Build history of the part. All positions in model axes, mm. Face numbers are marked on the shaded views. Coordinates: 2 decimals unless noted, no trailing zeros. Write each loop counter-clockwise with the first axis right and the second up, starting at its lowest first coordinate (ties: lowest second). Pieces come first, ordered by that corner, then holes.
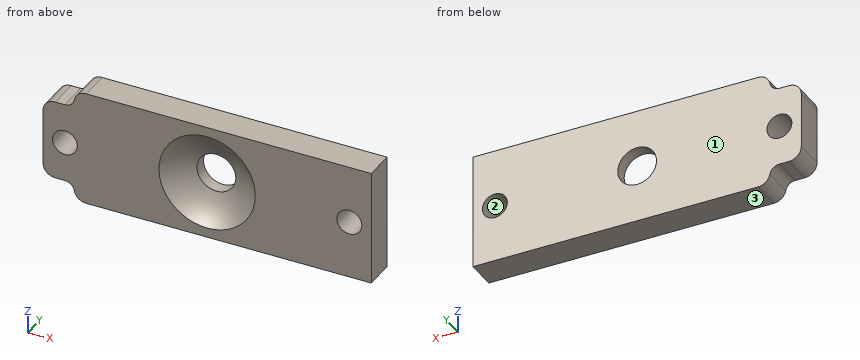
```python
from build123d import *

# Parameters (mm, degrees)
SKETCH2_W           = 68.58
SKETCH2_H           = 24.13
SKETCH2_R           = 2.6
BOSS_EXTRUDE1_DEPTH = 6.35
CUT_EXTRUDE1_DEPTH  = 7.35
FILLET3_R           = 2.54
SKETCH4_R           = 4.05
CUT_EXTRUDE2_DEPTH  = 7.3500001


with BuildPart() as part:
    # Sketch2 → Boss-Extrude1 (new body)
    with BuildSketch(Plane(origin=(0, 0, 0), x_dir=(1, 0, 0), z_dir=(0, 1, 0))):
        with Locations((34.29, 12.065)):
            Rectangle(SKETCH2_W, SKETCH2_H)
        with Locations((4.57, 12.065)):
            Circle(SKETCH2_R, mode=Mode.SUBTRACT)
        with Locations((64.01, 12.065)):
            Circle(SKETCH2_R, mode=Mode.SUBTRACT)
    extrude(amount=BOSS_EXTRUDE1_DEPTH)

    # Sketch3 → Cut-Extrude1 (cut, through all)
    with BuildSketch(Plane(origin=(0, 6.35, 0), x_dir=(1, 0, 0), z_dir=(0, 1, 0))):
        with BuildLine():
            Line((4.57, 3.715), (0, 3.715))
            Line((0, 3.715), (0, 0))
            Line((0, 0), (6.57, 0))
            Line((6.57, 0), (6.57, 1.715))
            ThreePointArc((6.57, 1.715), (5.984213562, 3.129213562), (4.57, 3.715))
        make_face()
        with BuildLine():
            ThreePointArc((4.57, 20.415), (5.984213562, 21.000786438), (6.57, 22.415))
            Line((6.57, 22.415), (6.57, 24.13))
            Line((6.57, 24.13), (0, 24.13))
            Line((0, 24.13), (0, 20.415))
            Line((0, 20.415), (4.57, 20.415))
        make_face()
    extrude(amount=-CUT_EXTRUDE1_DEPTH, mode=Mode.SUBTRACT)

    # Fillet3
    fillet3_edges = [part.edges().sort_by_distance(p)[0] for p in [
        (6.57, 3.175, 0),
        (0, 3.175, -3.715),
        (0, 3.175, -20.415),
        (6.57, 3.175, -24.13),
    ]]
    fillet(fillet3_edges, radius=FILLET3_R)

    # Sketch4 → Cut-Extrude2 (cut, through all)
    with BuildSketch(Plane(origin=(0, 6.35, 0), x_dir=(1, 0, 0), z_dir=(0, 1, 0))):
        with Locations((34.29, 12.065)):
            Circle(SKETCH4_R)
    extrude(amount=-CUT_EXTRUDE2_DEPTH, mode=Mode.SUBTRACT)

    # Sketch8 one side → Cut-Revolve6 (revolve, cut)
    with BuildSketch(Plane(origin=(34.29, 0, 0), x_dir=(0, 0, -1), z_dir=(1, 0, 0))):
        with BuildLine():
            Line((12.065, 0), (22.13, 0))
            ThreePointArc((22.13, 0), (17.5473974, 3.215969501), (12.065, 4.35))
            Line((12.065, 4.35), (12.065, 0))
        make_face()
    revolve(axis=Axis((34.29, 6.35, -12.065), (0, -1, 0)), mode=Mode.SUBTRACT)


solid = part.part
```
1. Probe line 1 along X through (y, z) = (6, -12); line 2 along X through (y, z) = (5, -12.75); line 3 along Z through (x, y) = (34.29, 5.3) (3 decimals). List the from-to ranges inside material, lowest first.
Computed values:
line 1: x = 0 to 1.97, 7.17 to 30.24, 38.34 to 61.41, 66.61 to 68.58
line 2: x = 0 to 2.06, 7.08 to 30.3, 38.28 to 61.5, 66.52 to 68.58
line 3: z = -24.13 to -16.115, -8.015 to 0
2. Saw through at B-B on x = 64.01. List the corners of the cut face in (y, z) (3 decimals), plus the area to 3 significant figures.
Computed values:
outline: (0, -24.13) - (6.35, -24.13) - (6.35, -14.665) - (0, -14.665) - close; (0, -9.465) - (6.35, -9.465) - (6.35, 0) - (0, 0) - close
area: 120 mm2
3. Saw through at C-C on y = 2.75. State how many separate pieces and enclosed holes the cut face has, plus the area to 3 significant figures.
Computed values:
separate pieces: 1
enclosed holes: 3
area: 1,430 mm2
4. Saw through at D-D on x = 43.5. List the corners of the cut face in (y, z) (3 decimals).
Computed values:
outline: (0, -24.13) - (6.35, -24.13) - (6.35, 0) - (0, 0) - (0, -8.005) arc R10.303 cw to (0, -16.125) - close
5. Flat gauge pins, fed straight in: pin 1 (9.5 mm diameter, centred on x = 34.29, z = -12.065, fed in from -Y); pin 2 (2 mm diameter, centred on x = 4, y = 2, fed in from -Z); pin 3 (1 mm diameter, centred on x = 4, y = 4, fed in from +Z) (3 decimals). Where does each tip first touch, or does it go through?
Computed values:
pin 1: stops at y = 3.51
pin 2: stops at z = -20.46
pin 3: stops at z = -3.715
6. Mould opens along Z. For the marked faces 1, 2 and 3 say: +Z half, -Z half, draft (parallel to the pull), parting line (faces both ways), or undercut.
Computed values:
face 1: draft
face 2: undercut
face 3: -Z half
7. Saw through at A-A on x = 34.29. List the corners of the cut face in (y, z) (3 decimals), plus the area to 3 significant figures.
Computed values:
outline: (0, -24.13) - (6.35, -24.13) - (6.35, -16.115) - (3.743, -16.115) arc R13.819 cw to (0, -22.13) - close; (0, -2) arc R13.819 cw to (3.743, -8.015) - (6.35, -8.015) - (6.35, 0) - (0, 0) - close
area: 74.9 mm2
